Geometry check sheet. Reference: drawing and pictorial views, mm from the part's lowest x, y, z. A direction names the side the tool comes from. Round coordinates to 2 decimals unless told otherwise and drop trailing zeros. Write each loop counter-clockwise with the first axis right and the second up, starting at its lowest first coordinate (ties: lowest second). Pieces come first, ordered by that corner, then holes. Notation, with made-up numbers: M 71.5,-1 L 101.5,-1 A17 ccw 101.5,22 Z; hole C -6.5,59 d11. An arc over 180 degrees is marked long. One line per item, written item: value. Start each with the question number.
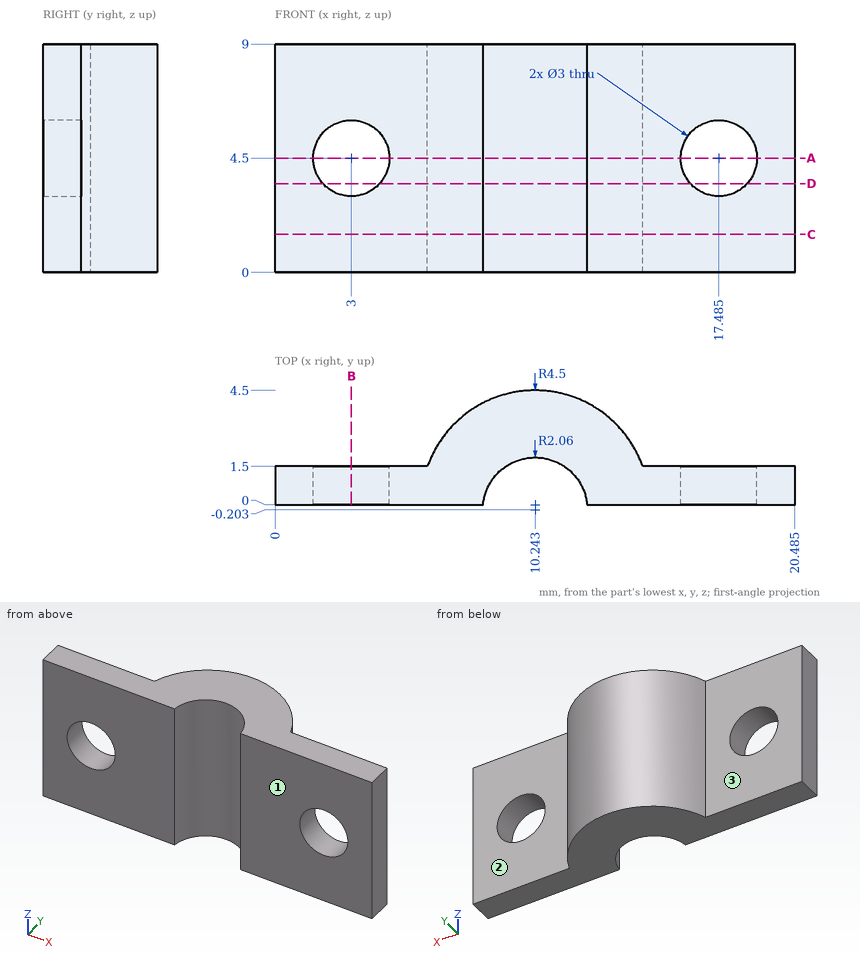
1) Thickness scan on line 1 (X direction, y = 0.9, z = 4.25) (1 decimal); line 2 (X direction, y = 1.35, z = 4) (1 decimal); line 3 (Y direction, x = 10.25, z = 8.5). Record the ranges inside material, lowest first.
2) Gauge pin test, flat ends, axial feed: pin 1 Ø1 at (x, z) = (3.5, 3.5) entering from +Y; pin 2 Ø1.8 at (x, z) = (17.49, 4.5) entering from -Y; pin 3 Ø2 at (x, z) = (10, 2.5) entering from -Y; pin 4 Ø2 at (y, z) = (3.5, 6.5) entering from +X (1 decimal). Record the tip position at first contact, or that the pin passes through.
3) Cross-section at B-B (x = 3). Record the boundary of the cut face in (y, z).
4) Access from +Z, -Z, +X, -X, +Y, -Y to the whole of each face (thin tool, end or side, straight path). Record for the marked faces 1, 2 and 3.
5) Cross-section at A-A (z = 4.5). Record the boundary of the cut face in (x, y) (1 decimal).
6) Cross-section at D-D (z = 3.5). Record the boundary of the cut face in (x, y) (1 decimal).
7) Cross-section at C-C (z = 1.5). Record the boundary of the cut face in (x, y) (1 decimal).
Results below:
1. line 1: x = 0 to 1.5, 4.5 to 8.5, 12 to 16, 19 to 20.5
1. line 2: x = 0 to 1.6, 4.4 to 8.9, 11.6 to 16.1, 18.9 to 20.5
1. line 3: y = 1.86 to 4.5
2. pin 1: stops at y = 1.5
2. pin 2: passes through
2. pin 3: stops at y = 1.44
2. pin 4: stops at x = 14
3. outline: M 0,0 L 1.5,0 L 1.5,3 L 0,3 Z; M 0,6 L 1.5,6 L 1.5,9 L 0,9 Z
4. face 1: +Z, -Z, +X, -X, -Y
4. face 2: +Z, -Z, +X, +Y
4. face 3: +Z, -Z, -X, +Y
5. outline: M 0,0 L 1.5,0 L 1.5,1.5 L 0,1.5 Z; M 4.5,0 L 8.2,0 A2.1 cw 12.3,0 L 16,0 L 16,1.5 L 14.5,1.5 A4.5 ccw 6,1.5 L 4.5,1.5 Z; M 19,0 L 20.5,0 L 20.5,1.5 L 19,1.5 Z
6. outline: M 0,0 L 1.9,0 L 1.9,1.5 L 0,1.5 Z; M 4.1,0 L 8.2,0 A2.1 cw 12.3,0 L 16.4,0 L 16.4,1.5 L 14.5,1.5 A4.5 ccw 6,1.5 L 4.1,1.5 Z; M 18.6,0 L 20.5,0 L 20.5,1.5 L 18.6,1.5 Z
7. outline: M 0,0 L 8.2,0 A2.1 cw 12.3,0 L 20.5,0 L 20.5,1.5 L 14.5,1.5 A4.5 ccw 6,1.5 L 0,1.5 Z
